Verification items for the finished model (mm, model axes). Face numbers are marked on the shaded views. Give positions to 0.01 mm unless a question says otherwise; leave off trailing zeros. Loops run counter-clockwise (first coordinate to the right, second up) from the corner with the lowest first, then second, coordinate; pieces in that order, holes last. Notation, with made-up numbers: M 53.5,76.5 L 71.5,76.5 A17 ccw 71.5,82.5 Z; hole C 46,59 d6. An arc over 180 degrees is marked long. Use a Markdown table: item, result.
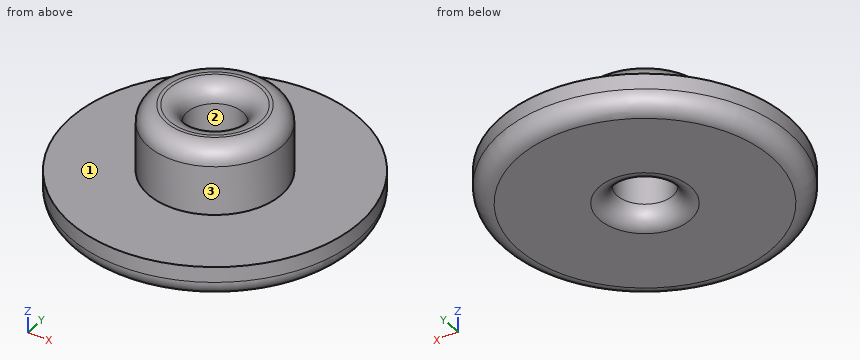
from build123d import *

# Parameters (mm, degrees)
F0_R     = 6.5
F1_DEPTH = 1.5
F2_R     = 3
F3_DEPTH = 3
F4_R     = 1.25
F5_DEPTH = 4.5
F6_R     = 0.8


with BuildPart() as f1:
    # F0 (on Top) → F1 (new body)
    with BuildSketch(Plane.XY):
        Circle(F0_R)
    extrude(amount=F1_DEPTH)

    # F2 (on face) → F3 (join)
    with BuildSketch(Plane.XY.offset(1.5)):
        Circle(F2_R)
    extrude(amount=F3_DEPTH)

    # F4 (on face) → F5 (cut, through all)
    with BuildSketch(Plane.XY.offset(4.5)):
        Circle(F4_R)
    extrude(amount=-F5_DEPTH, mode=Mode.SUBTRACT)

    # F6
    f6_edges = [f1.edges().sort_by_distance(p)[0] for p in [
        (-3, 0, 4.5),
        (-6.5, 0, 0),
        (-1.25, 0, 4.5),
        (-1.25, 0, 0),
    ]]
    fillet(f6_edges, radius=F6_R)


solid = f1.part
(1) Cross-section at A-A on y = 0. Record the cut outline in (x, z), then the cut area to 3 significant figures.
Results below:
| item | result |
|---|---|
| outline | M -6.5,0.8 A0.8 ccw -5.7,0 L -2.05,0 A0.8 ccw -1.25,0.8 L -1.25,3.7 A0.8 ccw -2.05,4.5 L -2.2,4.5 A0.8 ccw -3,3.7 L -3,1.5 L -6.5,1.5 Z; M 1.25,0.8 A0.8 ccw 2.05,0 L 5.7,0 A0.8 ccw 6.5,0.8 L 6.5,1.5 L 3,1.5 L 3,3.7 A0.8 ccw 2.2,4.5 L 2.05,4.5 A0.8 ccw 1.25,3.7 Z |
| area | 25.2 mm^2 |
(2) Draft check along Y on the marked faces 1, 2 and 3. Enter one of: +Y half, -Y half, draft (parallel to the pull), parting line (faces both ways), or undercut.
Results below:
| item | result |
|---|---|
| face 1 | draft |
| face 2 | undercut |
| face 3 | parting line |
(3) Material ranges on line 1 (Y direction, x = 0, z = 2.6); line 2 (Z direction, x = -2.25, y = -3.5); line 3 (X direction, y = -0.75, z = 3.3), recorded low to high.
Results below:
| item | result |
|---|---|
| line 1 | -3 to -1.25, 1.25 to 3 |
| line 2 | 0 to 1.5 |
| line 3 | -2.9 to -1, 1 to 2.9 |
(4) Cross-section at D-D on z = 2.8. Record the cut outline in (x, y), then the cut area to 3 significant figures.
Results below:
| item | result |
|---|---|
| outline | C 0,0 d6; hole C 0,0 d2.5 |
| area | 23.4 mm^2 |
(5) Cross-section at C-C on z = 1. Record the cut outline in (x, y).
Results below:
| item | result |
|---|---|
| outline | C 0,0 d13; hole C 0,0 d2.5 |
(6) Gauge pin test, flat ends, axial feed: P1, Ø1.5, axis at y = -4, z = 0.5, coming from the +X side; P2, Ø3, axis at x = 0.5, y = -4, coming from the +Z side; P3, Ø3, axis at x = 0, y = 0, coming from the +Z side. Record the tip position at first contact, or that the pin passes through.
Results below:
| item | result |
|---|---|
| P1 | x = 5.61 |
| P2 | z = 4.43 |
| P3 | z = 4.28 |
